```python
from build123d import *

# Parameters (mm, degrees)
SKETCH1_R           = 2.5
BOSS_EXTRUDE1_DEPTH = 30
CUT_EXTRUDE1_START  = -25
CUT_EXTRUDE1_DEPTH  = 25
SKETCH3_R           = 1.875
CUT_EXTRUDE2_DEPTH  = 128.328315782


with BuildPart() as part:
    # Sketch1 → Boss-Extrude1 (new body)
    with BuildSketch(Plane(origin=(0, 0, 0), x_dir=(1, 0, 0), z_dir=(0, 1, 0))):
        with BuildLine():
            Line((-10.853011104, 61.550484563), (-15.194215546, 86.170678389))
            ThreePointArc((-15.194215546, 86.170678389), (61.871843354, 61.871843354), (86.170678389, -15.194215546))
            Line((86.170678389, -15.194215546), (61.550484563, -10.853011104))
            ThreePointArc((61.550484563, -10.853011104), (44.194173824, 44.194173824), (-10.853011104, 61.550484563))
        make_face()
        with Locations(Location((75, 0, 0), (0, 0, 270))):
            Circle(SKETCH1_R, mode=Mode.SUBTRACT)
        with Locations(Location((0, 75, 0), (0, 0, 270))):
            Circle(SKETCH1_R, mode=Mode.SUBTRACT)
    extrude(amount=BOSS_EXTRUDE1_DEPTH)

    # Sketch2 → Cut-Extrude1 (cut)
    with BuildSketch(Plane(origin=(0, 30, 0), x_dir=(1, 0, 0), z_dir=(0, 1, 0)).offset(CUT_EXTRUDE1_START)):
        with BuildLine():
            Line((28.667524524, 55.537582209), (46.960542187, 73.830599872))
            ThreePointArc((46.960542187, 73.830599872), (61.871843354, 61.871843354), (73.830599872, 46.960542187))
            Line((73.830599872, 46.960542187), (55.537582209, 28.667524524))
            ThreePointArc((55.537582209, 28.667524524), (44.194173824, 44.194173824), (28.667524524, 55.537582209))
        make_face()
    extrude(amount=CUT_EXTRUDE1_DEPTH, mode=Mode.SUBTRACT)

    # Sketch3 → Cut-Extrude2 (cut, through all)
    with BuildSketch(Plane(origin=(0, 30, 0), x_dir=(1, 0, 0), z_dir=(0, 1, 0))):
        with Locations(Location((67.866071556, 34.63205284, 0), (0, 0, 270))):
            Circle(SKETCH3_R)
        with Locations(Location((34.63205284, 67.866071556, 0), (0, 0, 270))):
            Circle(SKETCH3_R)
    extrude(amount=-CUT_EXTRUDE2_DEPTH, mode=Mode.SUBTRACT)


solid = part.part
```
Model file for the job. Use its own axes, mm. A direction names the side the tool comes from. Round coordinates to 2 decimals unless told otherwise and drop trailing zeros. Write each loop counter-clockwise with the first axis right and the second up, starting at its lowest first coordinate (ties: lowest second). Pieces come first, ordered by that corner, then holes. Notation, with made-up numbers: (14, 62.5) - (44, 62.5) arc R12 ccw to (44, 83.5) - close; hole circle Ø8 at (46.5, 19). An arc over 180 degrees is marked (long way). One line per item, written item: value.
(1) Cut at A-A, the plane y = 11.75. Give the cut face in (x, z) (3 decimals), plus the area to 3 significant figures.
Values follow:
outline: (-15.194, -86.171) arc R87.5 ccw to (46.961, -73.831) - (28.668, -55.538) arc R62.5 cw to (-10.853, -61.55) - close; (55.538, -28.668) - (73.831, -46.961) arc R87.5 ccw to (86.171, 15.194) - (61.55, 10.853) arc R62.5 cw to start; hole circle Ø5 at (0, -75); hole circle Ø3.75 at (34.632, -67.866); hole circle Ø3.75 at (67.866, -34.632); hole circle Ø5 at (75, 0)
area: 2,580 mm²
(2) Cut at D-D, the plane z = -23. Give the cut face in (x, y).
Values follow:
outline: (58.11, 0) - (84.42, 0) - (84.42, 30) - (58.11, 30) - close
(3) Cut at B-B, the plane x = 0. Give the cut face in (y, z), plus the area to 3 significant figures.
Values follow:
outline: (0, -87.5) - (30, -87.5) - (30, -77.5) - (0, -77.5) - close; (0, -72.5) - (30, -72.5) - (30, -62.5) - (0, -62.5) - close
area: 600 mm²
(4) 3-axis set-ups, long thin cutter, end or side, ignore diameter. For faces 1 (the flat face through (37.69, 17.32, -64.56)), 2 (the flat face through (64.81, 17.32, -37.94)), 3 (the flat face through (52, 5, -52)): which of +Z, -Z, +X, -X, +Y, -Y reach the whole face in a straight line?
Values follow:
face 1: +Z, +X, +Y
face 2: -Z, -X, +Y
face 3: +Y
(5) Cut at C-C, the plane z = 0. Give the cut face in (x, y), plus the area to 3 significant figures.
Values follow:
outline: (62.5, 0) - (72.5, 0) - (72.5, 30) - (62.5, 30) - close; (77.5, 0) - (87.5, 0) - (87.5, 30) - (77.5, 30) - close
area: 600 mm²
(6) Two-plate mould, pull along Z, no slides. Class faces 4 (the cylindrical face through (44.78, 4.79, -43.6)), 5 (the flat face through (48, 0, -44)), 6 (the flat face through (74.033, 14.79, 13.054)): pulls with the +Z half, pulls with the -Z half, needs draft (parallel to the pull), parting line crosses it, or undercut.
Values follow:
face 4: undercut
face 5: needs draft
face 6: pulls with the +Z half
(7) Wall check: probe 1 along X at (y, z) = (19.5, 0); probe 2 along Z at (x, y) = (69, 2.5); probe 3 along X at (y, z) = (2.25, -33). Give the ranges that are in metal, low to high.
Values follow:
probe 1: x = 62.5 to 72.5, 77.5 to 87.5
probe 2: z = -53.81 to -36.13, -33.14 to 12.17
probe 3: x = 53.08 to 66.94, 68.79 to 81.04
(8) Drop flat-ended pins along their axis: P1, Ø8, axis at y = 19.5, z = -48, coming from the +X side; P2, Ø6, axis at x = 67.87, z = -34.63, coming from the +Y side; P3, Ø4, axis at x = 62.5, y = 15.5, coming from the +Z side; P4, Ø12, axis at x = 68, y = 21, coming from the +Z side. Give the stop position or say it passes through.
Values follow:
P1: stops at x = 75.63
P2: stops at y = 30
P3: stops at z = 11.37
P4: stops at z = 13.05
